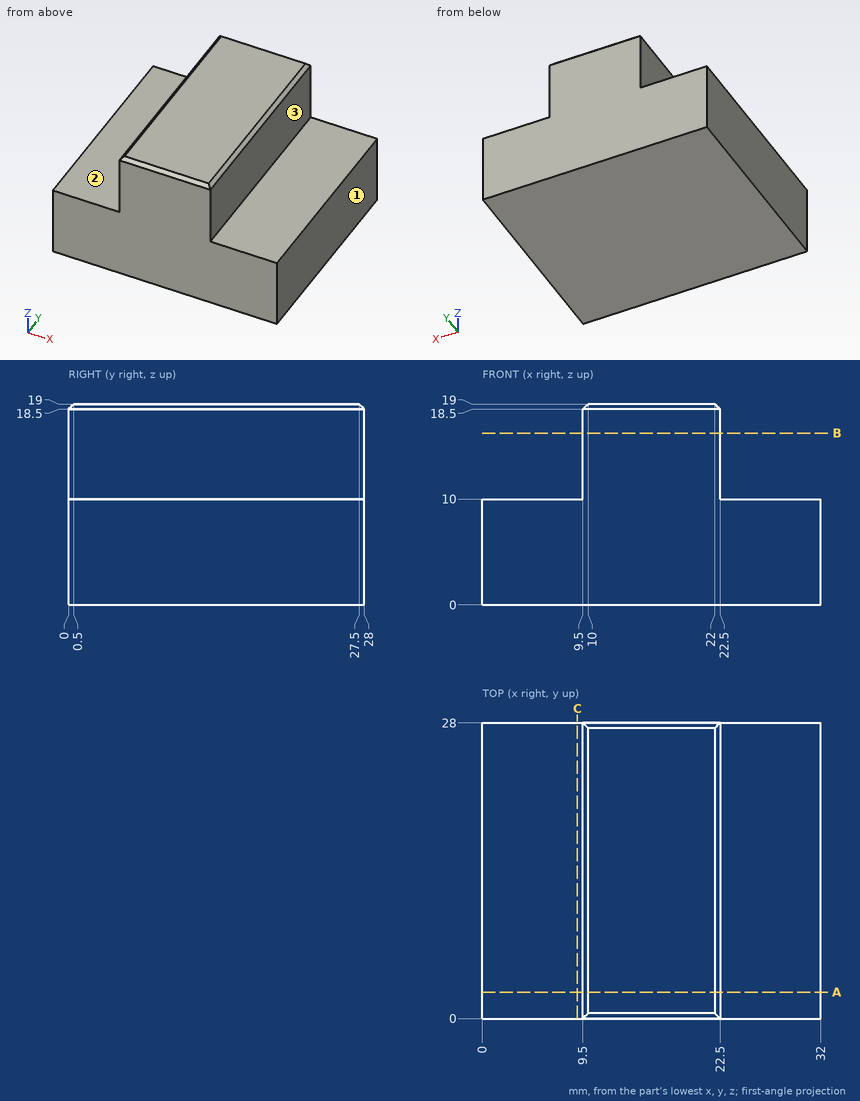
Design review of the part shown in the three views and the two pictorial views. Dimensions are in mm from the part's minimum x, y and z. A direction names the side the tool comes from. Round coordinates to 2 decimals unless told otherwise and drop trailing zeros. Loops run counter-clockwise (first coordinate to the right, second up) from the corner with the lowest first, then second, coordinate; pieces in that order, holes last. Notation, with made-up numbers: (2, 0) - (61, 0) arc R37 cw to (61, 36) - close; hole circle Ø6 at (-10, -33.75). An arc over 180 degrees is marked (long way). Write each question's results on one line, items separated by ' | '. Start each with the question number.
Q1. Take a section at A-A on y = 2.5. Give the boundary of the cut face in (x, z).
Q2. Tool access review of the marked faces 1, 2 and 3: name each direction out of +Z, -Z, +X, -X, +Y, -Y from which nothing blocks a thin tool from reaching the whole face with its end or side.
Q3. Take a section at C-C on x = 9. Give the boundary of the cut face in (y, z), plus the area to 3 significant figures.
Q4. Take a section at B-B on z = 16.25. Give the boundary of the cut face in (x, y), plus the area to 3 significant figures.
Q5. Wall thickness on line 1 along X through (y, z) = (15.5, 12); line 2 along Z through (x, y) = (26, 14.5): over which ranges is each line inside the solid? List them lowest first. Write a range as [from, to].
Q6. Insertion check: P1, Ø2.5, axis at y = 15.5, z = 15, coming from the +X side; P2, Ø7.5, axis at x = 28, y = 11, coming from the +Z side; P3, Ø2.5, axis at y = 7, z = 15, coming from the -X side. Each pin has a flat end and moves straight along its axis. Give the tip position at first contact, or say it passes through.
Data:
1) outline: (0, 0) - (32, 0) - (32, 10) - (22.5, 10) - (22.5, 18.5) - (22, 19) - (10, 19) - (9.5, 18.5) - (9.5, 10) - (0, 10) - close
2) face 1: +Z, -Z, +X, +Y, -Y | face 2: +Z, -X, +Y, -Y | face 3: +Z, +X, +Y, -Y
3) outline: (0, 0) - (28, 0) - (28, 10) - (0, 10) - close | area: 280 mm²
4) outline: (9.5, 0) - (22.5, 0) - (22.5, 28) - (9.5, 28) - close | area: 364 mm²
5) line 1: x = [9.5, 22.5] | line 2: z = [0, 10]
6) P1: stops at x = 22.5 | P2: stops at z = 10 | P3: stops at x = 9.5
